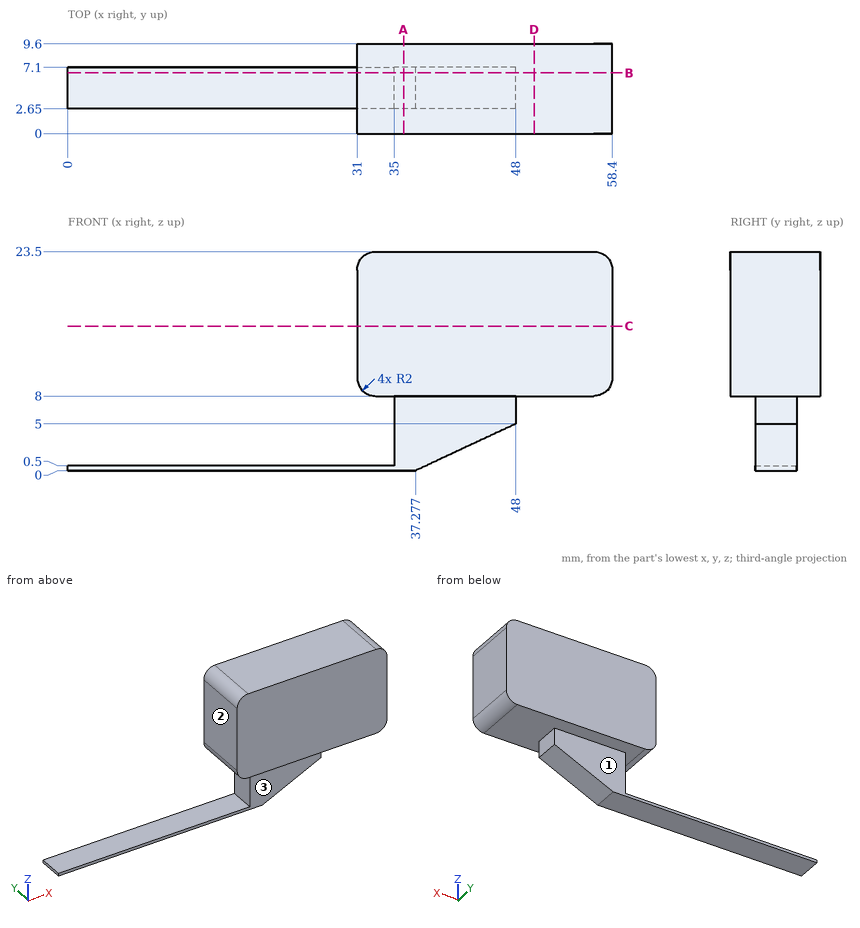
Answer from the drawing. Dimensions are ordinates in mm from the lowest x, y and z of the part. A direction names the side the tool comes from. Round coordinates to 2 decimals unless told otherwise and drop trailing zeros. Loops run counter-clockwise (first coordinate to the right, second up) from the corner with the lowest first, then second, coordinate; pieces in that order, holes last. Notation, with made-up numbers: M -5,15 L 13,15 A15 ccw 13,24 Z; hole C -9.5,-9 d3. An arc over 180 degrees is marked long. One line per question, with ' | ' between items. Start each with the question number.
(1) Find the intervals of material crossed by line 1 (X direction, y = 5.5, z = 16); line 2 (Z direction, x = 51.5, y = 1.75); line 3 (Z direction, x = 39.5, y = 3) (1 decimal), in increasing order.
(2) Flat-ended cylindrical pins translate along their axes: pin 1 Ø2 at (y, z) = (7.5, 11.5) entering from -X; pin 2 Ø2.5 at (y, z) = (4, 7) entering from +X; pin 3 Ø2 at (y, z) = (5, 4) entering from -X. Find the tip coordinate at first contact, or state that the pin passes through.
(3) A cutting plane is placed at A-A on x = 36. Write down the section's boundary in (y, z).
(4) A tool of negligible diameter and unlimited length cuts with its end or side. For the marked faces 1, 2 and 3, from which of +Z, -Z, +X, -X, +Y, -Y can it reach the whole face along a straight path? Write none if from no direction.
(5) A cutting plane is placed at B-B on y = 6.5. Write down the section's boundary in (x, z), plus the area to 3 significant figures.
(6) A cutting plane is placed at C-C on z = 15.5. Write down the section's boundary in (x, y), plus the area to 3 significant figures.
(7) A cutting plane is placed at D-D on x = 50. Write down the section's boundary in (y, z), plus the area to 3 significant figures.
Geometry check:
1) line 1: x = 31 to 58.4 | line 2: z = 8 to 23.5 | line 3: z = 1 to 23.5
2) pin 1: stops at x = 31 | pin 2: stops at x = 57.37 | pin 3: stops at x = 35
3) outline: M 0,8 L 2.65,8 L 2.65,0 L 7.1,0 L 7.1,8 L 9.6,8 L 9.6,23.5 L 0,23.5 Z
4) face 1: -Z, +X, -X, +Y | face 2: +Z, -X, +Y, -Y | face 3: -Z, +X, -X, -Y
5) outline: M 0,0 L 37.28,0 L 48,5 L 48,8 L 56.4,8 A2 ccw 58.4,10 L 58.4,21.5 A2 ccw 56.4,23.5 L 33,23.5 A2 ccw 31,21.5 L 31,10 A2 ccw 33,8 L 35,8 L 35,0.5 L 0,0.5 Z | area: 516 mm²
6) outline: M 31,0 L 58.4,0 L 58.4,9.6 L 31,9.6 Z | area: 263 mm²
7) outline: M 0,8 L 9.6,8 L 9.6,23.5 L 0,23.5 Z | area: 149 mm²
